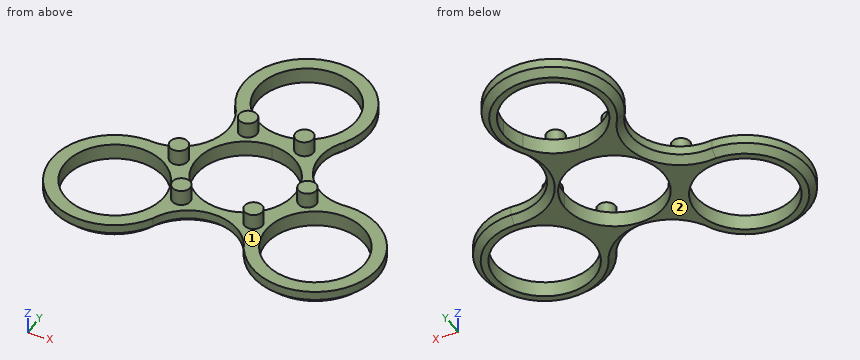
from build123d import *

# Parameters (mm, degrees)
F0_R       = 11
F0_R_2     = 2
F1_DEPTH   = 3.5
F2_DEPTH   = 7
F3_C1_SIZE = 1.5
F3_C2_SIZE = 1.5
F3_C3_SIZE = 1.5
F3_C4_SIZE = 1.5
F3_C5_SIZE = 1.5
F3_C6_SIZE = 1.5


with BuildPart() as f1:
    # F0 (on Top) → F1 (new body)
    with BuildSketch(Plane.XY):
        with BuildLine():
            ThreePointArc((22.164837833, 1.2031249106), (11.390396953, 6.576248747), (12.124355653, 18.5937501788))
            ThreePointArc((12.124355653, 18.5937501788), (0, 39.5937501788), (-12.124355653, 18.5937501788))
            ThreePointArc((-12.124355653, 18.5937501788), (-11.390396953, 6.576248747), (-22.164837833, 1.2031249106))
            ThreePointArc((-22.164837833, 1.2031249106), (-34.2891934859, -19.7968750894), (-10.04048218, -19.7968750894))
            ThreePointArc((-10.04048218, -19.7968750894), (0, -13.152497494), (10.04048218, -19.7968750894))
            ThreePointArc((10.04048218, -19.7968750894), (34.2891934859, -19.7968750894), (22.164837833, 1.2031249106))
        make_face()
        with Locations((-22.164837833, -12.7968750894)):
            Circle(F0_R, mode=Mode.SUBTRACT)
        with Locations((-7.9711980778, -11.7872301109)):
            Circle(F0_R_2, mode=Mode.SUBTRACT)
        with Locations((-14.1936397552, -1.0096449785)):
            Circle(F0_R_2, mode=Mode.SUBTRACT)
        with Locations((7.9711980778, -11.7872301109)):
            Circle(F0_R_2, mode=Mode.SUBTRACT)
        with Locations((22.164837833, -12.7968750894)):
            Circle(F0_R, mode=Mode.SUBTRACT)
        with BuildLine():
            ThreePointArc((0, 11), (7.7781745931, 7.7781745931), (11, 0))
            ThreePointArc((11, 0), (-7.7781745931, -7.7781745931), (0, 11))
        make_face(mode=Mode.SUBTRACT)
        with Locations((14.1936397552, -1.0096449785)):
            Circle(F0_R_2, mode=Mode.SUBTRACT)
        with Locations((-6.2224416774, 12.7968750894)):
            Circle(F0_R_2, mode=Mode.SUBTRACT)
        with Locations((6.2224416774, 12.7968750894)):
            Circle(F0_R_2, mode=Mode.SUBTRACT)
        with BuildLine():
            ThreePointArc((9.5262794416, 20.0937501788), (5.5, 16.0674707372), (0, 14.5937501788))
            ThreePointArc((0, 14.5937501788), (-5.5, 16.0674707372), (-9.5262794416, 20.0937501788))
            ThreePointArc((-9.5262794416, 20.0937501788), (-2.8470094961, 36.218934268), (11, 25.5937501788))
            ThreePointArc((11, 25.5937501788), (10.6251840892, 22.7467406827), (9.5262794416, 20.0937501788))
        make_face(mode=Mode.SUBTRACT)
    extrude(amount=F1_DEPTH)

    # F0 (on Top) → F2 (join)
    with BuildSketch(Plane.XY):
        with Locations((-6.2224416774, 12.7968750894)):
            Circle(F0_R_2)
        with Locations((6.2224416774, 12.7968750894)):
            Circle(F0_R_2)
        with Locations((14.1936397552, -1.0096449785)):
            Circle(F0_R_2)
        with Locations((7.9711980778, -11.7872301109)):
            Circle(F0_R_2)
        with Locations((-7.9711980778, -11.7872301109)):
            Circle(F0_R_2)
        with Locations((-14.1936397552, -1.0096449785)):
            Circle(F0_R_2)
    extrude(amount=F2_DEPTH)

    # F3: chamfer of 1.5 on 6 edges, made by hand

    # F3_c1
    f3_c1_edges = [f1.edges().sort_by_distance(p)[0] for p in [
        (0, -13.152497494, 0),
    ]]
    chamfer(f3_c1_edges, length=F3_C1_SIZE)

    # F3_c2
    f3_c2_edges = [f1.edges().sort_by_distance(p)[0] for p in [
        (11.390396953, 6.576248747, 0),
    ]]
    chamfer(f3_c2_edges, length=F3_C2_SIZE)

    # F3_c3
    f3_c3_edges = [f1.edges().sort_by_distance(p)[0] for p in [
        (-11.390396953, 6.576248747, 0),
    ]]
    chamfer(f3_c3_edges, length=F3_C3_SIZE)

    # F3_c4
    f3_c4_edges = [f1.edges().sort_by_distance(p)[0] for p in [
        (-34.2891934859, -19.7968750894, 0),
    ]]
    chamfer(f3_c4_edges, length=F3_C4_SIZE)

    # F3_c5
    f3_c5_edges = [f1.edges().sort_by_distance(p)[0] for p in [
        (34.2891934859, -19.7968750894, 0),
    ]]
    chamfer(f3_c5_edges, length=F3_C5_SIZE)

    # F3_c6
    f3_c6_edges = [f1.edges().sort_by_distance(p)[0] for p in [
        (0, 39.5937501788, 0),
    ]]
    chamfer(f3_c6_edges, length=F3_C6_SIZE)


solid = f1.part
Here's how the part is built. I have some questions about the finished solid (model axes, mm). Face numbers are marked on the shaded views. A direction names the side the tool comes from. Coordinates: 2 decimals unless noted, no trailing zeros. Loops run counter-clockwise (first coordinate to the right, second up) from the corner with the lowest first, then second, coordinate; pieces in that order, holes last.
1. For the marked faces 1 and 2, which set-ups out of +Z, -Z, +X, -X, +Y, -Y let a thin tool reach every point of the face, with its end or its side?
2. I need wall thicknesses on L1, parallel to X at y = -4.5, z = 1.5; L2, parallel to Z at x = -29.5, y = -22; L3, parallel to X at y = -21.5, z = 3. Which ranges of each line are inside material? Lowest first, please.
3. Imagine slicing it at A-A, the plane z = 5.5. Please give me the cut outline in (x, y).
4. Imagine slicing it at B-B, the plane x = -1.5. Count the separate pieces of the cut face and the enclosed holes in it, and give its area (3 significant figures).
5. For P1, Ø17.5, axis at x = -22.16, y = -12.8, coming from the -Z side; P2, Ø3, axis at x = -13, y = 5.5, coming from the +Z side; P3, Ø4, axis at x = 20, z = 2.5, coming from the -Y side, each with a flat end and sliding along its axis, tell me the tip position at first contact or that it passes through.
Taken from the geometry:
1. face 1: +Z
1. face 2: -Z, +X, -X, +Y, -Y
2. L1: x = -33.44 to -29.39, -14.94 to -10.04, 10.04 to 14.94, 29.39 to 33.44
2. L2: z = 0 to 3.5
2. L3: x = -33.13 to -28.89, -15.44 to -11.2, 11.2 to 15.44, 28.89 to 33.13
3. outline: circle Ø4 at (-14.19, -1.01); circle Ø4 at (-7.97, -11.79); circle Ø4 at (-6.22, 12.8); circle Ø4 at (6.22, 12.8); circle Ø4 at (7.97, -11.79); circle Ø4 at (14.19, -1.01)
4. separate pieces: 3
4. enclosed holes: 0
4. area: 29.9 mm2
5. P1: passes through
5. P2: stops at z = 3.5
5. P3: stops at y = -26.8
